Geometry check sheet. Reference: the model listing, model coordinates, mm. A direction names the side the tool comes from. Give positions to 0.01 mm unless a question says otherwise; leave off trailing zeros. One line per question, with ' | ' between items. Start each with the question number.
Q1. Section check A-A on z = 0.9. Count the separate pieces of the cut face and the enclosed holes in it, and give its area (3 significant figures).
Q2. Release check for a two-part mould opening along Y. For faces 1 (the face through (-19.04, 120.98, 1.48)), 2 (the face through (20.2, 63, 1)), 3 (the face through (-11.695, 149.178, 1.521)) record: +Y half, -Y half, draft (parallel to the pull), parting line (faces both ways), or undercut.
Q3. Set-up check for faces 4 (the face through (0, 75, 0)), 5 (the face through (-4.797, 106.341, 1.521)): record each of +Z, -Z, +X, -X, +Y, -Y from which the full face is reachable in a straight line by a thin tool's end or side.
Q4. Gauge pin test, flat ends, axial feed: P1, Ø2.5, axis at x = 11.5, y = 0, coming from the +Z side; P2, Ø1.5, axis at y = 128.5, z = 1.5, coming from the +X side; P3, Ø1.5, axis at x = 6, z = 1, coming from the +Y side. Record the tip position at first contact, or that the pin passes through.
Q5. Thickness scan on L1, parallel to Y at x = 11.5, z = 2.1; L2, parallel to Y at x = -9.5, z = 2.2; L3, parallel to Y at x = 9, z = 2.45. Record the ranges inside material, lowest first. Write a range as [from, to].
```python
from build123d import *

# Parameters (mm, degrees)
SKETCH1_R               = 7.95
SKETCH1_R_2             = 1.5
MAIN_BODY_LINK_B1_DEPTH = 3
CUT_EXTRUDE2_REACH      = 168.945
CUT_EXTRUDE3_REACH      = 168.945
SKETCH5_R               = 1.5
PULLEYIDLERUP_DEPTH     = 3
CUT_EXTRUDE5_DEPTH      = 3
FILLET4_R               = 1
FILLET5_R               = 100


with BuildPart() as part:
    # Sketch1 → Main Body Link B1 (new body)
    with BuildSketch(Plane.XY):
        with BuildLine():
            Line((20.2, 41.674052381), (20.2, 83.474052381))
            Line((20.2, 83.474052381), (20.2, 90.874052381))
            Line((20.2, 90.874052381), (17.986683974, 148.383116621))
            ThreePointArc((17.986683974, 148.383116621), (0, 165.690874165), (-17.986683974, 148.383116621))
            Line((-17.986683974, 148.383116621), (-20.2, 90.874052381))
            Line((-20.2, 90.874052381), (-20.2, 83.474052381))
            Line((-20.2, 83.474052381), (-20.2, 41.674052381))
            Line((-20.2, 41.674052381), (-20.2, 34.274052381))
            Line((-20.2, 34.274052381), (-17.964224051, -1.134307826))
            ThreePointArc((-17.964224051, -1.134307826), (0, -18), (17.964224051, -1.134307826))
            Line((17.964224051, -1.134307826), (20.2, 34.274052381))
            Line((20.2, 34.274052381), (20.2, 41.674052381))
        make_face()
        Circle(SKETCH1_R, mode=Mode.SUBTRACT)
        with Locations((15, 88.174052381)):
            Circle(SKETCH1_R_2, mode=Mode.SUBTRACT)
        with Locations((-15, 37.024052381)):
            Circle(SKETCH1_R_2, mode=Mode.SUBTRACT)
        with Locations((0, 147.690874165)):
            Circle(SKETCH1_R, mode=Mode.SUBTRACT)
    extrude(amount=MAIN_BODY_LINK_B1_DEPTH)

    # Sketch4 → Cut-Extrude2 (cut, up to next)
    with BuildSketch(Plane.XY.offset(3), mode=Mode.PRIVATE) as cut_extrude2_sk1:
        with BuildLine():
            Line((-12, 134.2744663), (-12, 123.584968066))
            Line((-12, 123.584968066), (-2.929911079, 129.930929878))
            ThreePointArc((-2.929911079, 129.930929878), (-7.774454217, 131.456408925), (-12, 134.2744663))
        make_face()
    cut_extrude2_tool1 = extrude(cut_extrude2_sk1.sketch, amount=-CUT_EXTRUDE2_REACH, mode=Mode.PRIVATE) & part.part
    # Sketch4 → Cut-Extrude2 (cut, up to next)
    with BuildSketch(Plane.XY.offset(3), mode=Mode.PRIVATE) as cut_extrude2_sk2:
        Polygon((-12, 100.690874165), (3.278172542, 100.690874165), (-12, 111.380372399), align=None)
    cut_extrude2_tool2 = extrude(cut_extrude2_sk2.sketch, amount=-CUT_EXTRUDE2_REACH, mode=Mode.PRIVATE) & part.part
    # Sketch4 → Cut-Extrude2 (cut, up to next)
    with BuildSketch(Plane.XY.offset(3), mode=Mode.PRIVATE) as cut_extrude2_sk3:
        Polygon((12, 128.172168466), (12, 106.793171999), (-3.278172542, 117.482670232), align=None)
    cut_extrude2_tool3 = extrude(cut_extrude2_sk3.sketch, amount=-CUT_EXTRUDE2_REACH, mode=Mode.PRIVATE) & part.part
    # Sketch4 → Cut-Extrude2 (cut, up to next)
    with BuildSketch(Plane.XY.offset(3), mode=Mode.PRIVATE) as cut_extrude2_sk4:
        Polygon((-4.386441158, 88.090874165), (12, 88.090874165), (12, 73.82101499), align=None)
    cut_extrude2_tool4 = extrude(cut_extrude2_sk4.sketch, amount=-CUT_EXTRUDE2_REACH, mode=Mode.PRIVATE) & part.part
    # Sketch4 → Cut-Extrude2 (cut, up to next)
    with BuildSketch(Plane.XY.offset(3), mode=Mode.PRIVATE) as cut_extrude2_sk5:
        Polygon((-12, 81.46073334), (-12, 52.92101499), (4.386441158, 67.190874165), align=None)
    cut_extrude2_tool5 = extrude(cut_extrude2_sk5.sketch, amount=-CUT_EXTRUDE2_REACH, mode=Mode.PRIVATE) & part.part
    # Sketch4 → Cut-Extrude2 (cut, up to next)
    with BuildSketch(Plane.XY.offset(3), mode=Mode.PRIVATE) as cut_extrude2_sk6:
        Polygon((-4.386441158, 46.290874165), (12, 46.290874165), (12, 60.56073334), align=None)
    cut_extrude2_tool6 = extrude(cut_extrude2_sk6.sketch, amount=-CUT_EXTRUDE2_REACH, mode=Mode.PRIVATE) & part.part
    add(cut_extrude2_tool1.solids().sort_by_distance((-9.12997, 128.978342, 3))[0], mode=Mode.SUBTRACT)
    add(cut_extrude2_tool2.solids().sort_by_distance((-6.907276, 104.25404, 3))[0], mode=Mode.SUBTRACT)
    add(cut_extrude2_tool3.solids().sort_by_distance((6.907276, 117.48267, 3))[0], mode=Mode.SUBTRACT)
    add(cut_extrude2_tool4.solids().sort_by_distance((6.537853, 83.334254, 3))[0], mode=Mode.SUBTRACT)
    add(cut_extrude2_tool5.solids().sort_by_distance((-6.537853, 67.190874, 3))[0], mode=Mode.SUBTRACT)
    add(cut_extrude2_tool6.solids().sort_by_distance((6.537853, 51.047494, 3))[0], mode=Mode.SUBTRACT)

    # Sketch5 → Cut-Extrude3 (cut, up to next)
    with BuildSketch(Plane.XY.offset(3), mode=Mode.PRIVATE) as cut_extrude3_sk1:
        with Locations((11.5, 147.690874165)):
            Circle(SKETCH5_R)
    cut_extrude3_tool1 = extrude(cut_extrude3_sk1.sketch, amount=-CUT_EXTRUDE3_REACH, mode=Mode.PRIVATE) & part.part
    # Sketch5 → Cut-Extrude3 (cut, up to next)
    with BuildSketch(Plane.XY.offset(3), mode=Mode.PRIVATE) as cut_extrude3_sk2:
        with Locations((-11.5, 147.690874165)):
            Circle(SKETCH5_R)
    cut_extrude3_tool2 = extrude(cut_extrude3_sk2.sketch, amount=-CUT_EXTRUDE3_REACH, mode=Mode.PRIVATE) & part.part
    # Sketch5 → Cut-Extrude3 (cut, up to next)
    with BuildSketch(Plane.XY.offset(3), mode=Mode.PRIVATE) as cut_extrude3_sk3:
        with Locations((-11.5, 0)):
            Circle(SKETCH5_R)
    cut_extrude3_tool3 = extrude(cut_extrude3_sk3.sketch, amount=-CUT_EXTRUDE3_REACH, mode=Mode.PRIVATE) & part.part
    # Sketch5 → Cut-Extrude3 (cut, up to next)
    with BuildSketch(Plane.XY.offset(3), mode=Mode.PRIVATE) as cut_extrude3_sk4:
        with Locations((11.5, 0)):
            Circle(SKETCH5_R)
    cut_extrude3_tool4 = extrude(cut_extrude3_sk4.sketch, amount=-CUT_EXTRUDE3_REACH, mode=Mode.PRIVATE) & part.part
    add(cut_extrude3_tool1.solids().sort_by_distance((11.5, 147.690874, 3))[0], mode=Mode.SUBTRACT)
    add(cut_extrude3_tool2.solids().sort_by_distance((-11.5, 147.690874, 3))[0], mode=Mode.SUBTRACT)
    add(cut_extrude3_tool3.solids().sort_by_distance((-11.5, 0, 3))[0], mode=Mode.SUBTRACT)
    add(cut_extrude3_tool4.solids().sort_by_distance((11.5, 0, 3))[0], mode=Mode.SUBTRACT)

    # Sketch6 → PulleyIdlerUp (cut)
    with BuildSketch(Plane.XY.offset(3)):
        with BuildLine():
            Line((-4.812543936, 110.623218529), (7.477908291, 102.024103222))
            ThreePointArc((7.477908291, 102.024103222), (9.566865044, 102.393236914), (9.197731352, 104.482193668))
            Line((9.197731352, 104.482193668), (-3.092720875, 113.081308975))
            ThreePointArc((-3.092720875, 113.081308975), (-5.181677628, 112.712175283), (-4.812543936, 110.623218529))
        make_face()
    extrude(amount=-PULLEYIDLERUP_DEPTH, mode=Mode.SUBTRACT)

    # Sketch7 → Cut-Extrude5 (cut)
    with BuildSketch(Plane.XY.offset(3)):
        with BuildLine():
            Line((-10.690189186, 25.65418917), (1.597091478, 17.050542625))
            ThreePointArc((1.597091478, 17.050542625), (3.686184199, 17.418906036), (3.317820787, 19.507998757))
            Line((3.317820787, 19.507998757), (-8.969459877, 28.111645303))
            ThreePointArc((-8.969459877, 28.111645303), (-11.058552598, 27.743281891), (-10.690189186, 25.65418917))
        make_face()
    extrude(amount=-CUT_EXTRUDE5_DEPTH, mode=Mode.SUBTRACT)

    # Fillet4
    fillet4_edges = [part.edges().sort_by_distance(p)[0] for p in [
        (-12, 81.46073334, 1.5),
        (4.386441158, 67.190874165, 1.5),
        (-12, 52.92101499, 1.5),
        (-12, 134.2744663, 1.5),
        (-2.929911079, 129.930929878, 1.5),
        (-12, 123.584968066, 1.5),
        (-12, 100.690874165, 1.5),
        (-12, 111.380372399, 1.5),
        (3.278172542, 100.690874165, 1.5),
        (12, 106.793171999, 1.5),
        (-3.278172542, 117.482670232, 1.5),
        (12, 128.172168466, 1.5),
        (12, 60.56073334, 1.5),
        (12, 46.290874165, 1.5),
        (-4.386441158, 46.290874165, 1.5),
        (12, 88.090874165, 1.5),
        (12, 73.82101499, 1.5),
        (-4.386441158, 88.090874165, 1.5),
    ]]
    fillet(fillet4_edges, radius=FILLET4_R)

    # Fillet5
    # the kernel refuses this fillet: 100 mm, written as the material it takes off along each edge
    with BuildSketch(Plane(origin=(-20.2, 34.274052381, -7.884973578), x_dir=(0, 1, 0), z_dir=(0, 0, 1))) as fillet5_piece_1:
        with BuildLine():
            CenterArc((FILLET5_R * 0.0315398943126, -FILLET5_R), FILLET5_R, 90, 3.613007947)
            Line((-FILLET5_R * 0.0314772071099, -FILLET5_R * 0.00198755271875), (0, 0))
            Line((0, 0), (FILLET5_R * 0.0315398943126, 0))
        make_face()
    extrude(amount=18.769947156, mode=Mode.SUBTRACT)
    with BuildSketch(Plane(origin=(-20.2, 90.874052381, -4.809018086), x_dir=(0.03845791424359976, 0.9992602207793684, 0), z_dir=(0, 0, 1))) as fillet5_piece_2:
        with BuildLine():
            CenterArc((FILLET5_R * 0.0192360723451, -FILLET5_R), FILLET5_R, 90, 2.204019698)
            Line((-FILLET5_R * 0.0192218418985, -FILLET5_R * 0.000739779220632), (0, 0))
            Line((0, 0), (FILLET5_R * 0.0192360723451, 0))
        make_face()
    extrude(amount=12.618036173, mode=Mode.SUBTRACT)
    with BuildSketch(Plane(origin=(20.2, 90.874052381, -4.809018086), x_dir=(-0.03845791424359111, 0.9992602207793686, 0), z_dir=(0, 0, 1))) as fillet5_piece_3:
        with BuildLine():
            CenterArc((FILLET5_R * 0.0192360723451, FILLET5_R), FILLET5_R, 267.795980302, 2.204019698)
            Line((-FILLET5_R * 0.0192218418985, FILLET5_R * 0.000739779220631), (0, 0))
            Line((0, 0), (FILLET5_R * 0.0192360723451, 0))
        make_face()
    extrude(amount=12.618036173, mode=Mode.SUBTRACT)
    with BuildSketch(Plane(origin=(20.2, 34.274052381, -7.884973578), x_dir=(0, 1, 0), z_dir=(0, 0, 1))) as fillet5_piece_4:
        with BuildLine():
            CenterArc((FILLET5_R * 0.0315398943126, FILLET5_R), FILLET5_R, 266.386992053, 3.613007947)
            Line((-FILLET5_R * 0.0314772071099, FILLET5_R * 0.00198755271875), (0, 0))
            Line((0, 0), (FILLET5_R * 0.0315398943126, 0))
        make_face()
    extrude(amount=18.769947156, mode=Mode.SUBTRACT)


solid = part.part
```
Working result:
1) separate pieces: 1 | enclosed holes: 16 | area: 5,500 mm2
2) face 1: +Y half | face 2: draft | face 3: undercut
3) face 4: -Z, +X, -X, +Y, -Y | face 5: +Z, -Z
4) P1: passes through | P2: stops at x = 18.78 | P3: stops at y = 164.91
5) L1: y = [-13.85, -1.5], [1.5, 46.42], [59.23, 75.15], [87.96, 107.85], [127.12, 146.19], [149.19, 161.54] | L2: y = [-15.29, 24.82], [28.35, 55.1], [79.28, 100.69], [109.63, 125.33], [132.4, 162.98] | L3: y = [-15.59, 46.29], [57.95, 76.43], [88.09, 101.91], [104.62, 108.89], [126.07, 163.28]
